```python
from build123d import *

# Parameters (mm, degrees)
SKETCH_W             = 36
SKETCH_H             = 18
PAD_DEPTH            = 8
POCKET_DEPTH         = 18.001
POCKET001_DEPTH      = 18.001
POCKET001_DEPTH_BACK = 18.001
FILLET_R             = 2
THICKNESS_T          = -1


with BuildPart() as part:
    # Sketch → Pad (new body)
    with BuildSketch(Plane.XY):
        Rectangle(SKETCH_W, SKETCH_H)
    extrude(amount=PAD_DEPTH)

    # Sketch001 (on Face1 of Pad) → Pocket (cut, through all)
    with BuildSketch(Plane.XZ.offset(9)):
        Polygon((-18, 8), (-18, 0), (-16, 8), align=None)
        Polygon((18, 8), (18, 0), (16, 8), align=None)
    extrude(amount=-POCKET_DEPTH, mode=Mode.SUBTRACT)

    # Sketch002 → Pocket001 (cut, two sides)
    with BuildSketch(Plane.YZ) as pocket001_sk:
        Polygon((-9, 8), (-7, 8), (-9, 0), align=None)
        Polygon((9, 8), (7, 8), (9, 0), align=None)
    extrude(amount=-POCKET001_DEPTH, mode=Mode.SUBTRACT)
    extrude(pocket001_sk.sketch, amount=POCKET001_DEPTH_BACK, mode=Mode.SUBTRACT)

    # Fillet
    fillet_edges = [part.edges().sort_by_distance(p)[0] for p in [
        (-17, 8, 4),
        (-17, -8, 4),
        (17, -8, 4),
        (17, 8, 4),
    ]]
    fillet(fillet_edges, radius=FILLET_R)

    # Thickness
    thickness_openings = [part.faces().sort_by_distance(p)[0] for p in [
        (0, 0, 0),
    ]]
    offset(amount=THICKNESS_T, openings=thickness_openings, kind=Kind.INTERSECTION)


solid = part.part
```
Verification items for the finished model (mm, model axes). A direction names the side the tool comes from. Give positions to 0.01 mm unless a question says otherwise; leave off trailing zeros. Write each loop counter-clockwise with the first axis right and the second up, starting at its lowest first coordinate (ties: lowest second). Pieces come first, ordered by that corner, then holes. Notation, with made-up numbers: M -28.5,25.25 L -23.5,25.25 A25 cw -23.5,37.25 Z; hole C 82.5,18 d7. An arc over 180 degrees is marked long. One line per question, with ' | ' between items.
1) Section check B-B on x = -2. Enter the section's corners in (y, z), plus the area to 3 significant figures.
Result:
outline: M -9,0 L -7.97,0 L -6.22,7 L 6.22,7 L 7.97,0 L 9,0 L 7,8 L -7,8 Z | area: 28.7 mm2
2) Set-up check for faces 1 (the flat face through (-16.106, -0.098, 3.451)), 2 (the cylindrical face through (-16.424, -7.454, 3.997)): record each of +Z, -Z, +X, -X, +Y, -Y from which the full face is reachable in a straight line by a thin tool's end or side.
Result:
face 1: -Z | face 2: +Z, -X, -Y
3) Thickness scan on line 1 along Z through (x, y) = (6, -5.5); line 2 along Y through (x, z) = (-11.5, 5); line 3 along Y through (x, z) = (-16, 0.75). Record the ranges inside material, lowest first. Write a range as [from, to].
Result:
line 1: z = [7, 8] | line 2: y = [-7.75, -6.72], [6.72, 7.75] | line 3: y = [-8.81, -7.76], [7.76, 8.81]
4) Mould release check, pull along Y, two halves, no side actions. Record for faces 3 (the cylindrical face through (16.425, -7.395, 4.112)), 4 (the cylindrical face through (-15.81, -6.82, 3.49)), 5 (the flat face through (0.22, 7.08, 3.55)), 6 (the cylindrical face through (-16.424, 7.454, 3.997)): released by +Y, released by -Y, zero draft, split by the parting line, or undercut.
Result:
face 3: released by -Y | face 4: undercut | face 5: undercut | face 6: released by +Y
5) Gauge pin test, flat ends, axial feed: pin 1 Ø2 at (x, z) = (13, 7) entering from +Y; pin 2 Ø2 at (x, z) = (-6, 3.5) entering from +Y (3 decimals); pin 3 Ø3 at (y, z) = (-1.5, 5) entering from +X (3 decimals). Record the tip position at first contact, or that the pin passes through.
Result:
pin 1: stops at y = 7.5 | pin 2: stops at y = 8.375 | pin 3: stops at x = 17.125
6) Section check A-A on y = 0.25. Enter the section's corners in (x, z), plus the area to 3 significant figures.
Result:
outline: M -18,0 L -16.97,0 L -15.22,7 L 15.22,7 L 16.97,0 L 18,0 L 16,8 L -16,8 Z | area: 46.7 mm2
